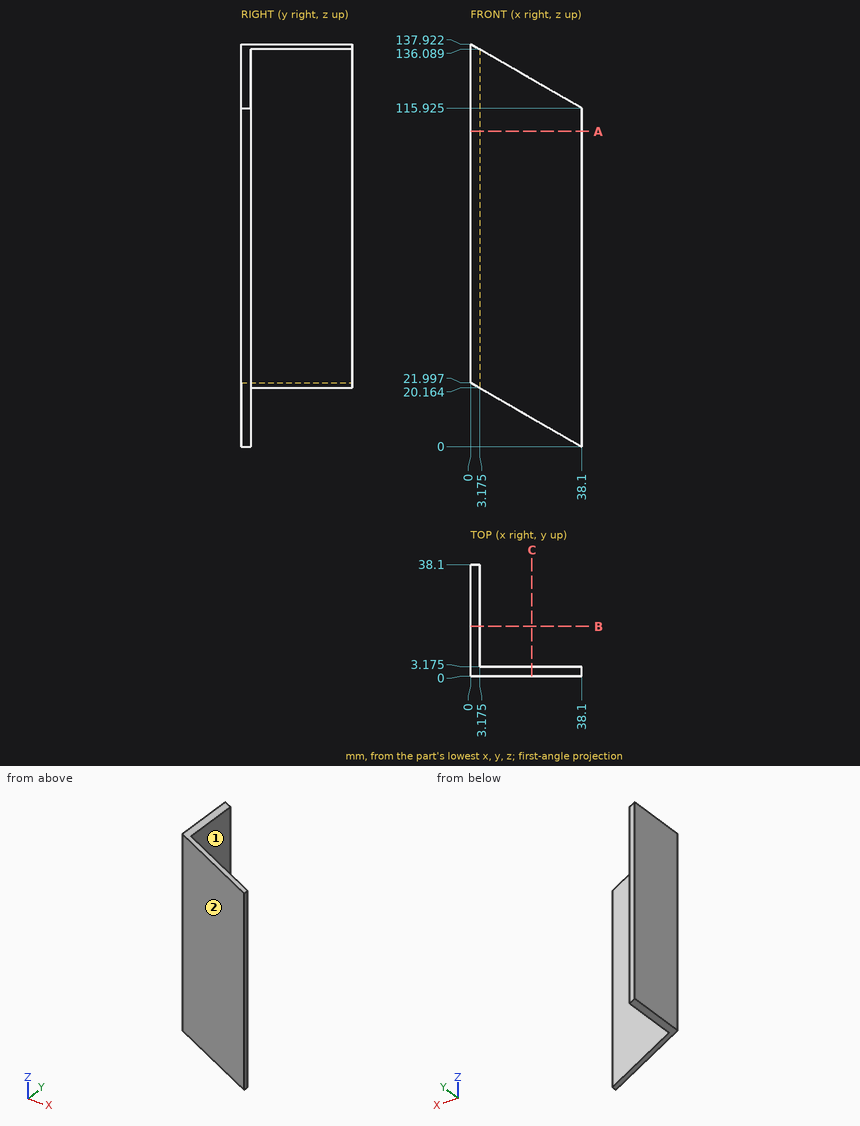
For this review, use the dimensioned drawing (mm, ordinates from the lowest corner) and the shaded views. A direction names the side the tool comes from. Round coordinates to 2 decimals unless told otherwise and drop trailing zeros. Order: outer loops, then holes, each group sorted by start corner. A loop starts at its lowest first (then second) coordinate and runs counter-clockwise, first axis right, second up. Notation, with made-up numbers: (69, 45) -> (119, 45) arc R21 ccw to (119, 49) -> close; hole circle Ø6 at (63, -14). An arc over 180 degrees is marked (long way). Put each result on its own line as item: value.
Q1. Add section A-A on z = 108. Write out the cut boundary in (x, y) (3 decimals).
Check result:
outline: (0, 0) -> (38.1, 0) -> (38.1, 3.175) -> (3.175, 3.175) -> (3.175, 38.1) -> (0, 38.1) -> close
Q2. Add section C-C on x = 21. Write out the cut boundary in (y, z) (1 decimal).
Check result:
outline: (0, 9.9) -> (3.2, 9.9) -> (3.2, 125.8) -> (0, 125.8) -> close
Q3. Insertion check: pin 1 Ø4 at (y, z) = (32.5, 36.5) entering from +X (3 decimals); pin 2 Ø17.5 at (x, z) = (19, 95) entering from +Y (3 decimals). Each pin has a flat end and moves straight along its axis. Give the tip position at first contact, or say it passes through.
Check result:
pin 1: x = 3.175
pin 2: y = 3.175
Q4. For probe 1 along Y at (x, z) = (21.5, 10) (3 decimals); probe 2 along Z at (x, y) = (16, 2.5), list the stretches that pass through material, from the lowest coordinate up. Write a range as [from, to].
Check result:
probe 1: [0, 3.175]
probe 2: [12.76, 128.68]
Q5. Add section B-B on y = 17. Write out the cut boundary in (x, z) (3 decimals).
Check result:
outline: (0, 21.997) -> (3.175, 20.164) -> (3.175, 136.089) -> (0, 137.922) -> close
Q6. Machinability: for the marked faces 1 and 2, which of the approach directions +Z, -Z, +X, -X, +Y, -Y give a long, thin tool a straight path to every point of the face, cutting with its end or side? Answer none if there is none.
Check result:
face 1: +Z, -Z, +X, +Y
face 2: +Z, -Z, +X, -X, -Y
